The model under review builds one solid part; all positions refer to its coordinate system, in mm. A direction names the side the tool comes from. Round coordinates to 2 decimals unless told otherwise and drop trailing zeros. Loops run counter-clockwise (first coordinate to the right, second up) from the corner with the lowest first, then second, coordinate; pieces in that order, holes last. Notation, with made-up numbers: M -37,68.5 L -23,68.5 A24 ccw -23,104.5 Z; hole C -22.75,54.5 d2. An arc over 180 degrees is marked long. Answer as a JSON object with one key per item and string values. Group by question number.
Item 1: The part is to be moulded in two halves that separate along X. For faces 1 (the face through (23.59, -5.72, 3.13)), 2 (the face through (19, -49, -6.35)), 3 (the face through (10.852, -30.34, 3.219)), 4 (the face through (104.14, -27, 3)), say which applies: +X half, -X half, draft (parallel to the pull), parting line (faces both ways), or undercut.
Item 2: Insertion check: P1, Ø1, axis at y = -26.5, z = 2, coming from the -X side; P2, Ø3.5, axis at x = 105.5, z = 3.5, coming from the +Y side; P3, Ø3, axis at y = -29, z = 3, coming from the -X side; P4, Ø4.5, axis at x = 19.05, y = -10.16, coming from the +Z side. Each pin has a flat end and moves straight along its axis. Give the tip position at first contact, or say it passes through.
Item 3: Consider section B-B (y = -32). Give the boundary of the cut face in (x, z) (3 decimals), and give its area (3 significant figures).
Item 4: Tool access review of faces 5 (the face through (12.993, -50.639, -1.5)), 6 (the face through (113.665, -33, 3)), 7 (the face through (103.416, -37.336, 3.131)): name each direction out of +Z, -Z, +X, -X, +Y, -Y from which nothing blocks a thin tool from reaching the whole face with its end or side.
Item 5: Consider section C-C (y = -46). Give the boundary of the cut face in (x, z).
Item 6: Consider section D-D (x = 91). Give the boundary of the cut face in (y, z), and give its area (3 significant figures).
Item 7: To check wall thickness, follow line 1 (Y direction, x = 19.05, z = 4) (3 decimals); line 2 (Y direction, x = 85, z = 5.5); line 3 (X direction, y = -37, z = 1.5) (3 decimals). State the ranges of each line that lie inside material, in increasing order.
Item 8: Consider section A-A (z = 5). Give the boundary of the cut face in (x, y) (3 decimals), and give its area (3 significant figures).
```python
from build123d import *

# Parameters (mm, degrees)
SKETCH1_R           = 1.905
BOSS_EXTRUDE1_DEPTH = 6.35
SKETCH3_R           = 6.35
BOSS_EXTRUDE2_DEPTH = 12.7
BOSS_EXTRUDE3_DEPTH = 6.35


with BuildPart() as part:
    # Sketch1 → Boss-Extrude1 (new body)
    with BuildSketch(Plane.XY):
        with BuildLine():
            Line((12.7, -10.16), (12.7, -48.731538364))
            ThreePointArc((12.7, -48.731538364), (14.760002182, -53.413249452), (19.603438966, -55.057374697))
            Line((19.603438966, -55.057374697), (107.868438966, -47.33518781))
            ThreePointArc((107.868438966, -47.33518781), (111.996711089, -45.299349296), (113.665, -41.009351478))
            Line((113.665, -41.009351478), (113.665, -25.4))
            ThreePointArc((113.665, -25.4), (111.805128061, -20.909871939), (107.315, -19.05))
            Line((107.315, -19.05), (104.14, -19.05))
            Line((104.14, -19.05), (104.14, -35.56))
            ThreePointArc((104.14, -35.56), (103.396051224, -37.356051224), (101.6, -38.1))
            Line((101.6, -38.1), (27.94, -38.1))
            ThreePointArc((27.94, -38.1), (26.143948776, -37.356051224), (25.4, -35.56))
            Line((25.4, -35.56), (25.4, -10.16))
            ThreePointArc((25.4, -10.16), (23.540128061, -5.669871939), (19.05, -3.81))
            ThreePointArc((19.05, -3.81), (14.559871939, -5.669871939), (12.7, -10.16))
        make_face()
        with Locations((19.05, -10.16)):
            Circle(SKETCH1_R, mode=Mode.SUBTRACT)
    extrude(amount=BOSS_EXTRUDE1_DEPTH)

    # Sketch3 → Boss-Extrude2 (add)
    with BuildSketch(Plane.XY.offset(6.35)):
        with Locations(Location((19.05, -48.731538364, 0), (0, 0, 180))):
            Circle(SKETCH3_R)
    extrude(amount=-BOSS_EXTRUDE2_DEPTH)

    # Sketch6 → Boss-Extrude3 (add)
    with BuildSketch(Plane.XY.offset(6.35)):
        with BuildLine():
            Line((12.730753591, -49.355737704), (8.920753591, -10.784199341))
            ThreePointArc((8.920753591, -10.784199341), (10.534356271, -5.896267235), (15.24, -3.81))
            Line((15.24, -3.81), (19.05, -3.81))
            ThreePointArc((19.05, -3.81), (14.559871939, -5.669871939), (12.7, -10.16))
            Line((12.7, -10.16), (12.7, -48.731538364))
            ThreePointArc((12.7, -48.731538364), (12.707693058, -49.044016603), (12.730753591, -49.355737704))
        make_face()
    extrude(amount=-BOSS_EXTRUDE3_DEPTH)


solid = part.part
```
Geometry results:
{
 "1": {"face 1": "+X half", "face 2": "draft", "face 3": "-X half", "face 4": "undercut"},
 "2": {"P1": "stops at x = 10.42", "P2": "stops at y = -19.05", "P3": "stops at x = 10.57", "P4": "stops at z = 6.35"},
 "3": {"outline": "M 11.016,0 L 25.4,0 L 25.4,6.35 L 11.016,6.35 Z; M 104.14,0 L 113.665,0 L 113.665,6.35 L 104.14,6.35 Z", "area": "152 mm^2"},
 "4": {"face 5": "-Z", "face 6": "+Z, -Z, +X, +Y, -Y", "face 7": "+Z, -Z, +Y"},
 "5": {"outline": "M 12.4,0 L 13.32,0 L 13.32,-6.35 L 24.78,-6.35 L 24.78,0 L 111.24,0 L 111.24,6.35 L 12.4,6.35 Z"},
 "6": {"outline": "M -48.81,0 L -38.1,0 L -38.1,6.35 L -48.81,6.35 Z", "area": "68.0 mm^2"},
 "7": {"line 1": "y = -55.082 to -12.065, -8.255 to -3.81", "line 2": "y = -49.34 to -38.1", "line 3": "x = 11.51 to 25.848, 103.692 to 113.665"},
 "8": {"outline": "M 8.921,-10.784 L 12.731,-49.356 A6.35 ccw 19.603,-55.057 L 107.868,-47.335 A6.35 ccw 113.665,-41.009 L 113.665,-25.4 A6.35 ccw 107.315,-19.05 L 104.14,-19.05 L 104.14,-35.56 A2.54 cw 101.6,-38.1 L 27.94,-38.1 A2.54 cw 25.4,-35.56 L 25.4,-10.16 A6.35 ccw 19.05,-3.81 L 15.24,-3.81 A6.35 ccw Z; hole C 19.05,-10.16 d3.81", "area": "1,990 mm^2"}
}
